Part print with two shaded views. Sizes in mm from the minimum x, y, z corner. A direction names the side the tool comes from. Round coordinates to 2 decimals unless told otherwise and drop trailing zeros. Order: outer loops, then holes, each group sorted by start corner. A loop starts at its lowest first (then second) coordinate and runs counter-clockwise, first axis right, second up. Notation, with made-up numbers: (-19.75, 43.25) - (23.25, 43.25) arc R27 ccw to (23.25, 79.25) - close; hole circle Ø1 at (11.25, 36). An arc over 180 degrees is marked (long way). Use one line per item in the form item = value.
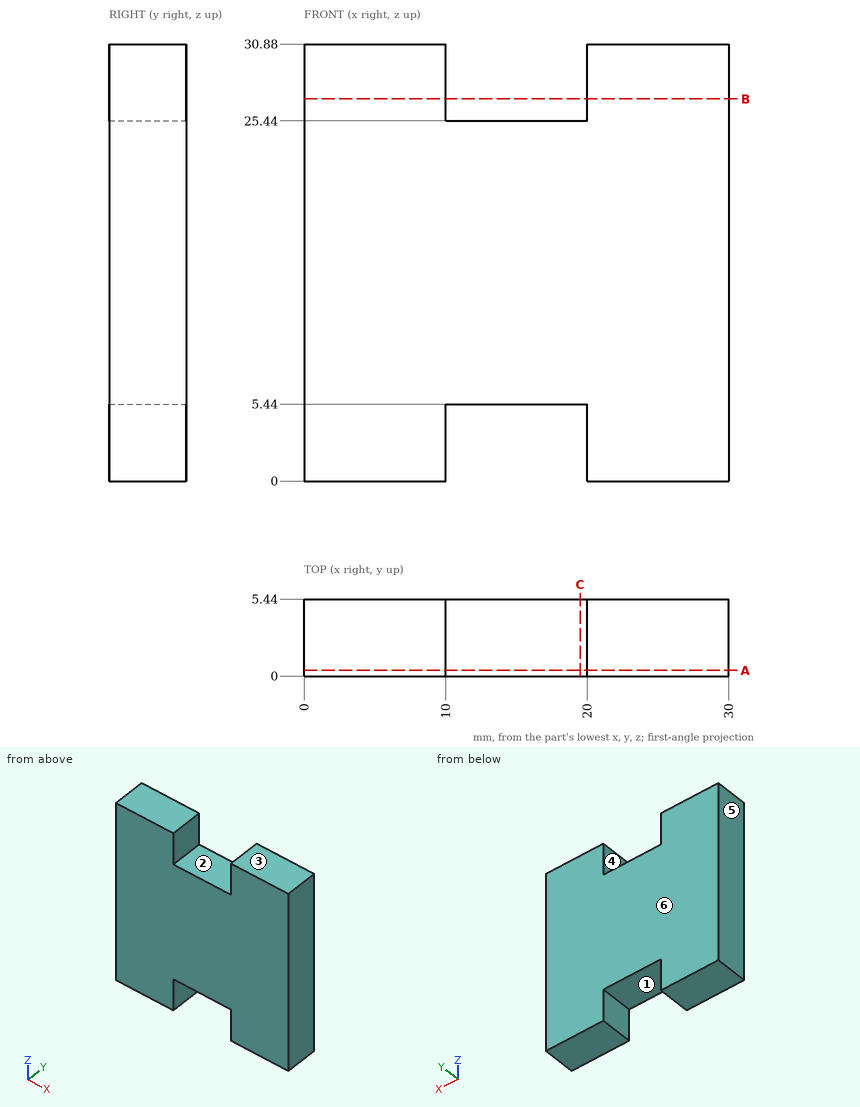
(1) Slice it at C-C on x = 19.5. Give the cut face in (y, z), then the cut area to 3 significant figures.
Report:
outline = (0, 5.44) - (5.44, 5.44) - (5.44, 25.44) - (0, 25.44) - close
area = 109 mm2
(2) Probe probe 1 along X at (y, z) = (3.85, 1.5); probe 2 along Z at (x, y) = (11, 0.95). List the from-to ranges inside material, lowest first. Write a range as [from, to].
Report:
probe_1 = [0, 10], [20, 30]
probe_2 = [5.44, 25.44]
(3) Slice it at B-B on z = 27. Give the cut face in (x, y).
Report:
outline = (0, 0) - (10, 0) - (10, 5.44) - (0, 5.44) - close; (20, 0) - (30, 0) - (30, 5.44) - (20, 5.44) - close
(4) Tool access for the marked faces 1, 2 and 3: list every direction of +Z, -Z, +X, -X, +Y, -Y with a clear straight run to the whole face (end or side of a thin tool).
Report:
face_1 = -Z, +Y, -Y
face_2 = +Z, +Y, -Y
face_3 = +Z, +X, -X, +Y, -Y
(5) Pull direction X, two halves, no side cores. Call the marked faces 4, 5 and 6: released by +X, released by -X, zero draft, split by the parting line, or undercut.
Report:
face_4 = undercut
face_5 = released by -X
face_6 = zero draft
(6) Slice it at A-A on y = 0.4. Give the cut face in (x, z).
Report:
outline = (0, 0) - (10, 0) - (10, 5.44) - (20, 5.44) - (20, 0) - (30, 0) - (30, 30.88) - (20, 30.88) - (20, 25.44) - (10, 25.44) - (10, 30.88) - (0, 30.88) - close
(7) Pin check, flat tips, straight feed: pin 1 (1.6 mm diameter, centred on x = 14.5, y = 2.5, fed in from -Z); pin 2 (2.5 mm diameter, centred on y = 2, z = 28, fed in from -X). Stop position of each tip, or through.
Report:
pin_1 = 5.44
pin_2 = 0
